```python
from build123d import *

# Parameters (mm, degrees)
BOSS_EXTRUDE1_DEPTH = 9
SKETCH3_R           = 1.5
BOSS_EXTRUDE2_DEPTH = 13.5
SKETCH2_R           = 1.5
BOSS_EXTRUDE3_DEPTH = 15


with BuildPart() as part:
    # Sketch1 → Boss-Extrude1 (new body)
    with BuildSketch(Plane.XY):
        with BuildLine():
            Line((-7.5, 27), (-4.5, 27))
            Line((-4.5, 27), (-4.5, 0))
            Line((-4.5, 0), (4.5, 0))
            Line((4.5, 0), (4.5, 27))
            Line((4.5, 27), (7.5, 27))
            Line((7.5, 27), (7.5, -0.221970842))
            ThreePointArc((7.5, -0.221970842), (8.110756434, -3.66320685), (9.868421053, -6.684091452))
            ThreePointArc((9.868421053, -6.684091452), (11.450319209, -9.402887593), (12, -12.5))
            Line((12, -12.5), (12, -36))
            Line((12, -36), (9, -36))
            Line((9, -36), (9, -12.5))
            ThreePointArc((9, -12.5), (6.363961031, -6.136038969), (0, -3.5))
            ThreePointArc((0, -3.5), (-6.363961031, -6.136038969), (-9, -12.5))
            Line((-9, -12.5), (-9, -36))
            Line((-9, -36), (-12, -36))
            Line((-12, -36), (-12, -12.5))
            ThreePointArc((-12, -12.5), (-11.450319209, -9.402887593), (-9.868421053, -6.684091452))
            ThreePointArc((-9.868421053, -6.684091452), (-8.110756434, -3.66320685), (-7.5, -0.221970842))
            Line((-7.5, -0.221970842), (-7.5, 27))
        make_face()
    extrude(amount=BOSS_EXTRUDE1_DEPTH)

    # Sketch3 → Boss-Extrude2 (add, symmetric)
    with BuildSketch(Plane(origin=(0, 0, 0), x_dir=(0, 0, -1), z_dir=(1, 0, 0))):
        with Locations((-4.5, -32)):
            Circle(SKETCH3_R)
    extrude(amount=BOSS_EXTRUDE2_DEPTH, both=True)

    # Sketch4 → Revolve1 (revolve)
    with BuildSketch(Plane.XY.offset(4.5)):
        with BuildLine():
            Line((-5, -32), (5, -32))
            Line((5, -32), (5, -17.590169944))
            ThreePointArc((5, -17.590169944), (0, -4.5), (-5, -17.590169944))
            Line((-5, -17.590169944), (-5, -32))
        make_face()
    revolve(axis=Axis((-13.5, -32, 4.5), (1, 0, 0)))

    # Sketch2 → Boss-Extrude3 (add)
    with BuildSketch(Plane(origin=(7.5, 0, 0), x_dir=(0, 0, -1), z_dir=(1, 0, 0))):
        with Locations((-4.5, 24)):
            Circle(SKETCH2_R)
        with Locations((-4.5, 8)):
            Circle(SKETCH2_R)
    extrude(amount=-BOSS_EXTRUDE3_DEPTH)


solid = part.part
```
Input: part model. Units: mm. Frame: model coordinates. A direction names the side the tool comes from. Coordinates: 2 decimals unless noted, no trailing zeros. Loops run counter-clockwise (first coordinate to the right, second up) from the corner with the lowest first, then second, coordinate; pieces in that order, holes last. Notation, with made-up numbers: (81, 47.5) - (113, 47.5) arc R14 ccw to (113, 63.5) - close; hole circle Ø10 at (78.5, 33.5). An arc over 180 degrees is marked (long way). Answer in a Markdown table with one row per item.
(1) Set-up query: faces 4 (the face through (0.063, 6.536, 4.825)), 5 (the face through (-1, -2, 0)), 6 (the face through (-10, -36, 4)). Return all of +Z, -Z, +X, -X, +Y, -Y with unobstructed straight access to the full face (end or side cutting, diameter ignored); none if empty.
Model answer:
| item | result |
|---|---|
| face 4 | none |
| face 5 | -Z, +Y |
| face 6 | +Z, -Z, -X, -Y |
(2) Mould query, pull axis Z, two halves, no side actions, for faces 1 (the face through (0, 0, 4)), 2 (the face through (0.063, 25.487, 4.695)), 3 (the face through (7, -32.9, 5.7)). Classes: pulls with the +Z half, pulls with the -Z half, needs draft (parallel to the pull), parting line crosses it, or undercut.
Model answer:
| item | result |
|---|---|
| face 1 | needs draft |
| face 2 | parting line crosses it |
| face 3 | undercut |
(3) Cut plane C-C on y = -32. Output: boundary loops of the cut face in (x, z), plus the area to 3 significant figures.
Model answer:
| item | result |
|---|---|
| outline | (-13.5, 3) - (-12, 3) - (-12, 0) - (-9, 0) - (-9, 3) - (-5, 3) - (-5, -9.91) arc R7.5 ccw (long way) to (5, -9.91) - (5, 3) - (9, 3) - (9, 0) - (12, 0) - (12, 3) - (13.5, 3) - (13.5, 6) - (12, 6) - (12, 9) - (9, 9) - (9, 6) - (5, 6) - (5, 18.91) arc R7.5 ccw (long way) to (-5, 18.91) - (-5, 6) - (-9, 6) - (-9, 9) - (-12, 9) - (-12, 6) - (-13.5, 6) - close |
| area | 702 mm² |
(4) Cut plane D-D on z = 4.5. Count the separate pieces of the cut face and the enclosed holes in it, plus the area to 3 significant figures.
Model answer:
| item | result |
|---|---|
| separate pieces | 1 |
| enclosed holes | 3 |
| area | 1,120 mm² |
(5) Pin query (flat end, axial travel): P1, Ø0.9, axis at x = 11, z = 6.5, coming from the -Y side; P2, Ø6, axis at y = -37.5, z = 4.5, coming from the +X side; P3, Ø1.5, axis at x = -6.5, z = 19, coming from the +Y side. Return the tip coordinate at first contact, or that it passes through.
Model answer:
| item | result |
|---|---|
| P1 | stops at y = -36 |
| P2 | stops at x = 12 |
| P3 | stops at y = -11.74 |
(6) Cut plane B-B on x = 2.5. Output: boundary loops of the cut face in (y, z), plus the area to 3 significant figures.
Model answer:
| item | result |
|---|---|
| outline | circle Ø54.14 at (-32, 4.5); (-3.85, 0) - (0, 0) - (0, 9) - (-3.85, 9) - close; circle Ø3 at (8, 4.5); circle Ø3 at (24, 4.5) |
| area | 2,350 mm² |
(7) Material intervals for L1, parallel to X at y = -32.5, z = 8; L2, parallel to X at y = -16, z = 1.5; L3, parallel to Z at x = -11.5, y = -21, sorted ascending. Write a range as from..to.
Model answer:
| item | result |
|---|---|
| L1 | x = -12..-9, -5..5, 9..12 |
| L2 | x = -12..-9, -6.51..6.51, 9..12 |
| L3 | z = 0..9 |
(8) Cut plane A-A on y = 19.5. Output: boundary loops of the cut face in (x, z), plus the area to 3 significant figures.
Model answer:
| item | result |
|---|---|
| outline | (-7.5, 0) - (-4.5, 0) - (-4.5, 9) - (-7.5, 9) - close; (4.5, 0) - (7.5, 0) - (7.5, 9) - (4.5, 9) - close |
| area | 54.0 mm² |
